```python
from build123d import *

# Parameters (mm, degrees)
BOSS_EXTRUDE1_DEPTH          = 21.59
SHELL3_T                     = -2.54
SKETCH2_R                    = 3.175
PIN_HOLES_DEPTH              = 195.673850517
SKETCH3_R                    = 6.35
TOW_HITCH_ADAPTOR_HOLE_DEPTH = 22.59


with BuildPart() as part:
    # Sketch1 → Boss-Extrude1 (new body)
    with BuildSketch(Plane(origin=(0, 0, 0), x_dir=(1, 0, 0), z_dir=(0, 1, 0))):
        Polygon((0, 0), (-609.6, 0), (-914.4, 175.976362049), (-903.605, 194.673850517), (-603.814976935, 21.59), (0, 21.59), align=None)
    extrude(amount=-BOSS_EXTRUDE1_DEPTH)

    # Shell3
    shell3_openings = [part.faces().sort_by_distance(p)[0] for p in [
        (-909.0025, -10.795, -185.325106283),
        (0, -10.795, -10.795),
    ]]
    offset(amount=SHELL3_T, openings=shell3_openings, kind=Kind.INTERSECTION)

    # Sketch2 → PIN HOLES (cut, through all)
    with BuildSketch(Plane.XY):
        with Locations((-120.65, -10.791269693)):
            Circle(SKETCH2_R)
        with Locations((-31.75, -10.791269693)):
            Circle(SKETCH2_R)
    extrude(amount=-PIN_HOLES_DEPTH, mode=Mode.SUBTRACT)

    # Sketch3 → TOW HITCH ADAPTOR HOLE (cut, through all)
    with BuildSketch(Plane(origin=(0, 0, 0), x_dir=(1, 0, 0), z_dir=(0, 1, 0))):
        with Locations((-897.686477372, 179.525032414)):
            Circle(SKETCH3_R)
    extrude(amount=-TOW_HITCH_ADAPTOR_HOLE_DEPTH, mode=Mode.SUBTRACT)


solid = part.part
```
Here's how the part is built. I have some questions about the finished solid (model axes, mm). A direction names the side the tool comes from. Coordinates: 2 decimals unless noted, no trailing zeros. Order: outer loops, then holes, each group sorted by start corner. A loop starts at its lowest first (then second) coordinate and runs counter-clockwise, first axis right, second up.
1) Will these pins go through, and if not, where does the flat tip stop? pin 1 (3 mm diameter, centred on x = -244.5, y = -18, fed in from -Z); pin 2 (3 mm diameter, centred on y = -18, z = -109.5, fed in from +X); pin 3 (12 mm diameter, centred on y = -8, z = -169, fed in from -X).
2) We'd pull the mould along Z, two halves only. Please class faces 5 (the face through (-759.87, -10.64, -86.76)), 6 (the face through (-455, 0, -18)), 7 (the face through (-488, -19.05, -14)): +Z half, -Z half, draft (parallel to the pull), parting line (faces both ways), or undercut.
3) I need wall thicknesses on line 1 (Y direction, x = -354, z = -17); line 2 (Y direction, x = -120.65, z = -20.65). Which ranges of each line are inside material? Lowest first, please.
4) Imagine slicing it at A-A on x = -382. List the corners of the cut face in (y, z) for me, and give its area (3 significant figures).
5) Imagine slicing it at B-B on z = -75.5. List the corners of the cut face in (x, y) for me, and give its area (3 significant figures).
6) Which directions (+Z, -Z, +X, -X, +Y, -Y) give clear straight access to the entire face, cutting with the end or side of a thin tool? Please do faces 1 (the face through (-455, -21.59, -18)), 2 (the face through (-306, -11, -21.59)), 3 (the face through (-758.9, -10.68, -89.13)), 4 (the face through (-306, -11, -19.05)).
Response values:
1. pin 1: stops at z = -21.59
1. pin 2: stops at x = -753.48
1. pin 3: stops at x = -912.71
2. face 5: +Z half
2. face 6: draft
2. face 7: undercut
3. line 1: y = -21.59 to -19.05, -2.54 to 0
3. line 2: y = -21.59 to -13.97, -7.62 to 0
4. outline: (-21.59, -21.59) - (0, -21.59) - (0, 0) - (-21.59, 0) - close; hole (-19.05, -19.05) - (-2.54, -19.05) - (-2.54, -2.54) - (-19.05, -2.54) - close
4. area: 194 mm2
5. outline: (-740.37, -21.59) - (-697.19, -21.59) - (-697.19, 0) - (-740.37, 0) - close; hole (-735.29, -19.05) - (-702.27, -19.05) - (-702.27, -2.54) - (-735.29, -2.54) - close
5. area: 387 mm2
6. face 1: +Z, -Z, +X, -X, -Y
6. face 2: -Z, +X, +Y, -Y
6. face 3: none
6. face 4: +X
